Check sheet for the modelled part. Datum: model origin and axes. Units: mm. Face numbers are marked on the shaded views. A direction names the side the tool comes from. Give positions to 0.01 mm unless a question says otherwise; leave off trailing zeros. Order: outer loops, then holes, each group sorted by start corner. A loop starts at its lowest first (then second) coordinate and runs counter-clockwise, first axis right, second up.
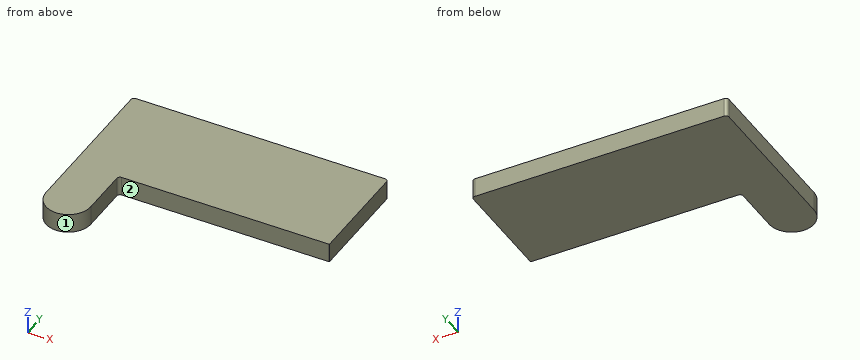
```python
from build123d import *

# Parameters (mm, degrees)
BODY_DEPTH = 1.5


with BuildPart() as part:
    # Sketch1 → Body (new body, symmetric)
    with BuildSketch(Plane.XY):
        with BuildLine():
            Line((0, 0), (0, 24.5))
            ThreePointArc((0, 24.5), (0.146446609, 24.853553391), (0.5, 25))
            Line((0.5, 25), (28.339745962, 25))
            Line((28.339745962, 25), (39.5, 25))
            ThreePointArc((39.5, 25), (39.853553391, 24.853553391), (40, 24.5))
            Line((40, 24.5), (40, 8.1))
            ThreePointArc((40, 8.1), (39.970710678, 8.029289322), (39.9, 8))
            Line((39.9, 8), (36.966924922, 8))
            Line((36.966924922, 8), (7.5, 8))
            ThreePointArc((7.5, 8), (7.146446609, 7.853553391), (7, 7.5))
            Line((7, 7.5), (7, 0))
            ThreePointArc((7, 0), (3.5, -3.5), (0, 0))
        make_face()
    extrude(amount=BODY_DEPTH, both=True)


solid = part.part
```
(1) Gauge pin test, flat ends, axial feed: pin 1 Ø1.5 at (x, z) = (35, 0) entering from -Y; pin 2 Ø0.9 at (y, z) = (2.5, -0.5) entering from +X. Record the tip position at first contact, or that the pin passes through.
Response values:
pin 1: stops at y = 8
pin 2: stops at x = 7
(2) Cross-section at A-A on z = -0.4. Enter the section's corners in (x, y), then the cut area to 3 significant figures.
Response values:
outline: (0, 0) arc R3.5 ccw to (7, 0) - (7, 7.5) arc R0.5 cw to (7.5, 8) - (39.9, 8) arc R0.1 ccw to (40, 8.1) - (40, 24.5) arc R0.5 ccw to (39.5, 25) - (0.5, 25) arc R0.5 ccw to (0, 24.5) - close
area: 755 mm2
(3) Material ranges on L1, parallel to X at y = 4, z = -0.6; L2, parallel to Y at x = 27, z = 0.85; L3, parallel to Y at x = 2, z = -1.1, recorded low to high.
Response values:
L1: x = 0 to 7
L2: y = 8 to 25
L3: y = -3.16 to 25
(4) Cross-section at B-B on y = 3.25. Enter the section's corners in (x, z).
Response values:
outline: (0, -1.5) - (7, -1.5) - (7, 1.5) - (0, 1.5) - close
(5) Set-up check for the marked faces 1 and 2: record each of +Z, -Z, +X, -X, +Y, -Y from which the full face is reachable in a straight line by a thin tool's end or side.
Response values:
face 1: +Z, -Z, -Y
face 2: +Z, -Z, +X, -Y
(6) Cross-section at C-C on x = 32.5. Enter the section's corners in (y, z).
Response values:
outline: (8, -1.5) - (25, -1.5) - (25, 1.5) - (8, 1.5) - close
